Here's how the part is built. I have some questions about the finished solid (model axes, mm). A direction names the side the tool comes from. Coordinates: 2 decimals unless noted, no trailing zeros. Loops run counter-clockwise (first coordinate to the right, second up) from the corner with the lowest first, then second, coordinate; pieces in that order, holes last. Notation, with made-up numbers: (-24.75, 78.25) -> (26.25, 78.25) arc R20 cw to (26.25, 92.25) -> close; hole circle Ø6 at (87, 49). An arc over 180 degrees is marked (long way). Answer as a JSON object with one key per item and string values. Group by question number.
1) If we mould it in two halves opening along Z, with no side actions, what happens to faces 3 (the flat face through (123, 0, -103)), 4 (the cylindrical face through (127.884, 1.565, -102.378))? For each: +Z half, -Z half, draft (parallel to the pull), parting line (faces both ways), or undercut.
2) I want a section at C-C (z = -101.6). Count the separate pieces of the cut face and the enclosed holes in it, then the cut area to 3 significant figures.
3) Which directions (+Z, -Z, +X, -X, +Y, -Y) give clear straight access to the entire face, cutting with the end or side of a thin tool? Please do faces 1 (the cylindrical face through (92.165, 1.565, -123)), 2 (the flat face through (95, 2.286, -102)).
4) I need wall thicknesses on probe 1 along Z at (x, y) = (158.75, 2.05); probe 2 along X at (y, z) = (2.3, -158.75); probe 3 along Z at (x, y) = (101.6, 2.9). Which ranges of each line are inside material? Lowest first, please. Write a range as [from, to].
5) I want a section at B-B (x = 44.45). Write out the boundary of the cut face in (y, z) (3 decimals), then the cut area to 3 significant figures.
6) I'm going to push a flat-ended pin straight in: pin 1 (7.5 mm diameter, centred on x = 15.93, z = -101.6, fed in from +Y) (3 decimals). Where does the tip first touch, or does it pass through?
7) I want a section at A-A (z = -158.75). Write out the boundary of the cut face in (x, y) (3 decimals).
```python
from build123d import *

# Parameters (mm, degrees)
SKETCH1_W           = 203.2
SKETCH1_H           = 203.2
SKETCH1_R           = 2.45745
SKETCH1_R_2         = 2.5908
SKETCH1_R_3         = 2.413
BOSS_EXTRUDE1_DEPTH = 3.175
SKETCH2_R           = 14.2875
CUT_EXTRUDE1_DEPTH  = 0.889


with BuildPart() as part:
    # Sketch1 → Boss-Extrude1 (new body)
    with BuildSketch(Plane(origin=(0, 0, 0), x_dir=(1, 0, 0), z_dir=(0, 1, 0))):
        with Locations((101.6, 101.6)):
            Rectangle(SKETCH1_W, SKETCH1_H)
        with Locations((44.45, 158.75)):
            Circle(SKETCH1_R, mode=Mode.SUBTRACT)
        with Locations((44.45, 101.6)):
            Circle(SKETCH1_R, mode=Mode.SUBTRACT)
        with Locations((44.45, 44.45)):
            Circle(SKETCH1_R, mode=Mode.SUBTRACT)
        with Locations((158.75, 44.45)):
            Circle(SKETCH1_R, mode=Mode.SUBTRACT)
        with Locations((158.75, 101.6)):
            Circle(SKETCH1_R, mode=Mode.SUBTRACT)
        with Locations((158.75, 158.75)):
            Circle(SKETCH1_R, mode=Mode.SUBTRACT)
        with Locations((77.7875, 101.6)):
            Circle(SKETCH1_R_2, mode=Mode.SUBTRACT)
        with Locations((89.69375, 122.222229928)):
            Circle(SKETCH1_R_2, mode=Mode.SUBTRACT)
        with Locations((89.69375, 80.977770072)):
            Circle(SKETCH1_R_2, mode=Mode.SUBTRACT)
        with Locations((113.50625, 122.222229928)):
            Circle(SKETCH1_R_2, mode=Mode.SUBTRACT)
        with Locations((125.4125, 101.6)):
            Circle(SKETCH1_R_2, mode=Mode.SUBTRACT)
        with Locations((113.50625, 80.977770072)):
            Circle(SKETCH1_R_2, mode=Mode.SUBTRACT)
        with Locations((101.6, 187.271643395)):
            Circle(SKETCH1_R_3, mode=Mode.SUBTRACT)
        with Locations((187.271643395, 101.6)):
            Circle(SKETCH1_R_3, mode=Mode.SUBTRACT)
        with Locations((101.6, 15.928356605)):
            Circle(SKETCH1_R_3, mode=Mode.SUBTRACT)
        with Locations((15.928356605, 101.6)):
            Circle(SKETCH1_R_3, mode=Mode.SUBTRACT)
        Polygon((107.95, 105.266174209), (101.6, 108.932348419), (95.25, 105.266174209), (95.25, 97.933825791), (101.6, 94.267651581), (107.95, 97.933825791), align=None, mode=Mode.SUBTRACT)
    extrude(amount=BOSS_EXTRUDE1_DEPTH)

    # Sketch2 → Cut-Extrude1 (cut)
    with BuildSketch(Plane(origin=(0, 3.175, 0), x_dir=(1, 0, 0), z_dir=(0, 1, 0))):
        with Locations((101.6, 101.6)):
            Circle(SKETCH2_R)
    extrude(amount=-CUT_EXTRUDE1_DEPTH, mode=Mode.SUBTRACT)


solid = part.part
```
Determined:
{
 "1": {"face 3": "draft", "face 4": "undercut"},
 "2": {"separate pieces": "8", "enclosed holes": "0", "area": "496 mm^2"},
 "3": {"face 1": "+Y, -Y", "face 2": "+Y"},
 "4": {"probe 1": "[-203.2, -161.21], [-156.29, -104.06], [-99.14, -46.91], [-41.99, 0]", "probe 2": "[0, 41.99], [46.91, 156.29], [161.21, 203.2]", "probe 3": "[-203.2, -189.68], [-184.86, -115.89], [-87.31, -18.34], [-13.52, 0]"},
 "5": {"outline": "(0, -203.2) -> (3.175, -203.2) -> (3.175, -161.207) -> (0, -161.207) -> close; (0, -156.293) -> (3.175, -156.293) -> (3.175, -104.057) -> (0, -104.057) -> close; (0, -99.143) -> (3.175, -99.143) -> (3.175, -46.907) -> (0, -46.907) -> close; (0, -41.993) -> (3.175, -41.993) -> (3.175, 0) -> (0, 0) -> close", "area": "598 mm^2"},
 "6": {"pin 1": "y = 3.175"},
 "7": {"outline": "(0, 0) -> (41.993, 0) -> (41.993, 3.175) -> (0, 3.175) -> close; (46.907, 0) -> (156.293, 0) -> (156.293, 3.175) -> (46.907, 3.175) -> close; (161.207, 0) -> (203.2, 0) -> (203.2, 3.175) -> (161.207, 3.175) -> close"}
}
